Can you work these out from the model? Positions are in its coordinate system, mm. A direction names the side the tool comes from. Coordinates: 2 decimals unless noted, no trailing zeros. Order: outer loops, then holes, each group sorted by start corner. A loop starts at its lowest first (then second) coordinate and runs counter-clockwise, first axis right, second up. Notation, with made-up numbers: (18.5, -10) - (72.5, -10) arc R20 ccw to (72.5, 15) - close; hole circle Ø1 at (-11.5, 80.25). An arc over 180 degrees is marked (long way). Use a Markdown table: item, result. Add a question column.
(1) We'd pull the mould along X, two halves only. Please class faces 1 (the flat face through (0.1, 6, 2.3)), 2 (the cylindrical face through (-0.2, 0.8, 5.3)), 3 (the cylindrical face through (-1.081, 3.782, 3.434)): pulls with the +X half, pulls with the -X half, needs draft (parallel to the pull), parting line crosses it, or undercut.
(2) I want a section at B-B (z = -4.8). List the corners of the cut face in (x, y) for me.
(3) On a 3-axis mill with a long thin cutter (end or side, diameter ignored), from which of +Z, -Z, +X, -X, +Y, -Y can I reach the whole of each face in a straight line? I mean faces 4 (the flat face through (3, 1.5, 3)), 5 (the flat face through (0, 0, 3)), 6 (the flat face through (0, 3, 1.9)). Say none if no direction works.
(4) I want a section at A-A (x = 0). List the corners of the cut face in (y, z) for me.
(5) I want a section at C-C (y = 0.85). List the corners of the cut face in (x, z) for me.
(6) For pin 1 Ø4 at (x, z) = (4, -1.5) entering from -Y; pin 2 Ø1.1 at (y, z) = (3, -1) entering from +X; pin 3 Ø1.6 at (x, y) = (1, 3) entering from -Z; pin 4 Ø1.4 at (x, z) = (4.8, 0) entering from +Y, each with a flat end and sliding along its axis, tell me the tip position at first contact or that it passes through.
(7) I want a section at D-D (x = 4.8). List the corners of the cut face in (y, z) for me.
(8) If I drill on L1, parallel to X at y = 0.75, z = 0; L2, parallel to Y at x = 3.25, z = 3.5; L3, parallel to X at y = 0.6, z = -4.8, over which ranges is the centre line in solid material (lowest first)? Write a range as [from, to].
```python
from build123d import *

# Parameters (mm, degrees)
SKETCH1_R           = 6
SKETCH1_W           = 5.3
SKETCH1_H           = 3.8
BOSS_EXTRUDE1_DEPTH = 6
SKETCH6_W           = 2.4
SKETCH6_H           = 4.5
SKETCH10_R          = 0.54
CUT_EXTRUDE2_DEPTH  = 60


with BuildPart() as part:
    # Sketch1 → Boss-Extrude1 (new body)
    with BuildSketch(Plane(origin=(0, 0, 0), x_dir=(1, 0, 0), z_dir=(0, 1, 0))):
        with Locations(Location((0, 0, 0), (0, 0, 270))):
            Circle(SKETCH1_R)
        Rectangle(SKETCH1_W, SKETCH1_H, mode=Mode.SUBTRACT)
    extrude(amount=BOSS_EXTRUDE1_DEPTH)

    # Sketch6 → Cut-Revolve1 (revolve, cut)
    with BuildSketch(Plane(origin=(0, 0, 0), x_dir=(0, 0, -1), z_dir=(1, 0, 0))):
        with Locations((-4.8, 3.75)):
            Rectangle(SKETCH6_W, SKETCH6_H)
    revolve(axis=Axis((0, 6, 0), (0, -1, 0)), mode=Mode.SUBTRACT)

    # Sketch10 → Cut-Extrude2 (cut)
    with BuildSketch(Plane(origin=(0, 1.5, 0), x_dir=(1, 0, 0), z_dir=(0, 1, 0))):
        with Locations(Location((-4.8, 0, 0), (0, 0, 270))):
            Circle(SKETCH10_R)
        with Locations(Location((0, -4.8, 0), (0, 0, 270))):
            Circle(SKETCH10_R)
        with Locations(Location((4.8, 0, 0), (0, 0, 270))):
            Circle(SKETCH10_R)
        with Locations(Location((0, 4.8, 0), (0, 0, 270))):
            Circle(SKETCH10_R)
    extrude(amount=-CUT_EXTRUDE2_DEPTH, mode=Mode.SUBTRACT)


solid = part.part
```
Answers follow:
| question | item | result |
|---|---|---|
| 1 | face 1 | needs draft |
| 1 | face 2 | undercut |
| 1 | face 3 | parting line crosses it |
| 2 | outline | (-3.6, 0) - (-0.54, 0) - (-0.54, 1.5) - (-3.6, 1.5) - close; (0.54, 0) - (3.6, 0) - (3.6, 1.5) - (0.54, 1.5) - close |
| 3 | face 4 | +Y |
| 3 | face 5 | +Z, -Z, +X, -X, -Y |
| 3 | face 6 | +Y, -Y |
| 4 | outline | (0, -6) - (1.5, -6) - (1.5, -5.34) - (0, -5.34) - close; (0, -4.26) - (1.5, -4.26) - (1.5, -3.6) - (6, -3.6) - (6, -1.9) - (0, -1.9) - close; (0, 1.9) - (6, 1.9) - (6, 3.6) - (1.5, 3.6) - (1.5, 4.26) - (0, 4.26) - close; (0, 5.34) - (1.5, 5.34) - (1.5, 6) - (0, 6) - close |
| 5 | outline | circle Ø12 at (0, 0); hole circle Ø1.08 at (-4.8, 0); hole (-2.65, -1.9) - (2.65, -1.9) - (2.65, 1.9) - (-2.65, 1.9) - close; hole circle Ø1.08 at (0, -4.8); hole circle Ø1.08 at (0, 4.8); hole circle Ø1.08 at (4.8, 0) |
| 6 | pin 1 | stops at y = 0 |
| 6 | pin 2 | stops at x = 3.57 |
| 6 | pin 3 | stops at z = -3.59 |
| 6 | pin 4 | stops at y = 1.5 |
| 7 | outline | (0, -3.6) - (1.5, -3.6) - (1.5, -0.54) - (0, -0.54) - close; (0, 0.54) - (1.5, 0.54) - (1.5, 3.6) - (0, 3.6) - close |
| 8 | L1 | x = [-6, -5.34], [-4.26, -2.65], [2.65, 4.26], [5.34, 6] |
| 8 | L2 | y = [0, 1.5] |
| 8 | L3 | x = [-3.6, -0.54], [0.54, 3.6] |
